Design review of the part built by this model. Coordinates are the model's own, in mm. A direction names the side the tool comes from. Round coordinates to 2 decimals unless told otherwise and drop trailing zeros. Loops run counter-clockwise (first coordinate to the right, second up) from the corner with the lowest first, then second, coordinate; pieces in that order, holes last. Notation, with made-up numbers: (-21.5, 88.25) - (17.5, 88.25) arc R15 cw to (17.5, 95.25) - close; hole circle Ø10 at (-14, -38.5). An arc over 180 degrees is marked (long way). Return JSON: item names as keys, results as strings. Group by question number.
from build123d import *

# Parameters (mm, degrees)
SKETCH3_R           = 2.5
BOSS_EXTRUDE1_DEPTH = 4.15
SKETCH4_R           = 1.5
BOSS_EXTRUDE2_DEPTH = 2
SKETCH4_3_R         = 1.5
BOSS_EXTRUDE3_DEPTH = 2
SKETCH4_5_R         = 1.5
BOSS_EXTRUDE4_DEPTH = 4.15
BOSS_EXTRUDE5_DEPTH = 2
CIRPATTERN1_COUNT   = 32


with BuildPart() as part:
    # Sketch3 → Boss-Extrude1 (new body)
    with BuildSketch(Plane(origin=(0, 0, 0), x_dir=(1, 0, 0), z_dir=(0, 1, 0))):
        with Locations(Location((0, 0, 0), (0, 0, 90))):
            Circle(SKETCH3_R)
    extrude(amount=BOSS_EXTRUDE1_DEPTH)

    # Sketch4 → Boss-Extrude2 (add)
    with BuildSketch(Plane(origin=(0, 4.15, 0), x_dir=(1, 0, 0), z_dir=(0, 1, 0))):
        with BuildLine():
            Line((30, 4), (10.915155748, 4))
            ThreePointArc((10.915155748, 4), (-11.625, 0), (10.915155748, -4))
            Line((10.915155748, -4), (30, -4))
            ThreePointArc((30, -4), (34, 0), (30, 4))
        make_face()
        with Locations(Location((30, 0, 0), (0, 0, 270))):
            Circle(SKETCH4_R, mode=Mode.SUBTRACT)
    extrude(amount=BOSS_EXTRUDE2_DEPTH)

    # Sketch4<3> → Boss-Extrude3 (add)
    with BuildSketch(Plane(origin=(0, 4.15, 0), x_dir=(1, 0, 0), z_dir=(0, 1, 0))):
        with Locations((30, 0)):
            Circle(SKETCH4_3_R)
    extrude(amount=BOSS_EXTRUDE3_DEPTH)

    # Sketch4<5> → Boss-Extrude4 (add)
    with BuildSketch(Plane(origin=(0, 4.15, 0), x_dir=(1, 0, 0), z_dir=(0, 1, 0))):
        with Locations(Location((30, 0, 0), (0, 0, 270))):
            Circle(SKETCH4_5_R)
    extrude(amount=-BOSS_EXTRUDE4_DEPTH)

    # Sketch7 → Boss-Extrude5 (add)
    with BuildSketch(Plane(origin=(0, 6.15, 0), x_dir=(1, 0, 0), z_dir=(0, 1, 0))):
        Polygon((-11.366268694, 0.75), (-11.366268694, -0.75), (-13.166268694, -0.25), (-13.166268694, 0.25), align=None)
    boss_extrude5 = extrude(amount=-BOSS_EXTRUDE5_DEPTH)

    # CirPattern1: Boss-Extrude5 ×32 about axis
    cirpattern1_axis = Axis((0, 0, 0), (0, 1, 0))
    for i in range(1, CIRPATTERN1_COUNT):
        add(boss_extrude5.rotate(cirpattern1_axis, i * 360 / CIRPATTERN1_COUNT))


solid = part.part
Q1. Draft analysis for pull direction X (two halves, no side actions). For faces 1 (the flat face through (8.418, 5.164, -9.082)), 2 (the flat face through (0, 0, 0)), 3 (the flat face through (-12.045, 5.164, 2.875)), state which applies: pulls with the +X half, pulls with the -X half, needs draft (parallel to the pull), parting line crosses it, or undercut.
Q2. Insertion check: pin 1 Ø2 at (x, y) = (19, 5.5) entering from -Z; pin 2 Ø3 at (y, z) = (4, -6) entering from +X; pin 3 Ø1.5 at (x, z) = (2, -5) entering from -Y. Each pin has a flat end and moves straight along its axis. Give the tip position at first contact, or say it passes through.
Q3. Add section B-B, the plane x = 18.5. State the section outline as (y, z) points, plus the area to 3 significant figures.
Q4. For line 1 (Z direction, x = 11.5, y = 5.5); line 2 (X direction, y = 4.5, z = -12); line 3 (X direction, y = 5.25, z = -10.5), list the stretches that pass through material, from the lowest coordinate up.
Q5. Add section A-A, the plane y = 1.25. State the section outline as (x, z) points.
Q6. Tool access review of faces 4 (the cylindrical face through (-11.123, 5.136, -3.381)), 5 (the flat face through (6.484, 5.164, -10.55)), 6 (the flat face through (1.964, 5.164, 12.249)), 7 (the flat face through (11.275, 5.164, 5.172)): name each direction out of +Z, -Z, +X, -X, +Y, -Y from which nothing blocks a thin tool from reaching the whole face with its end or side.
Evaluation:
{
 "1": {"face 1": "undercut", "face 2": "needs draft", "face 3": "pulls with the -X half"},
 "2": {"pin 1": "z = -4", "pin 2": "x = 12.26", "pin 3": "y = 4.15"},
 "3": {"outline": "(4.15, -4) - (6.15, -4) - (6.15, 4) - (4.15, 4) - close", "area": "16.0 mm²"},
 "4": {"line 1": "-5.2 to -4.21, -4 to 4, 4.21 to 5.2", "line 2": "-5.26 to -4.6, -2.88 to -1.84, -0.57 to 0.57, 1.84 to 2.88, 4.6 to 5.26", "line 3": "-7.42 to -6.43, -5.08 to 5.08, 6.43 to 7.42"},
 "5": {"outline": "circle Ø5 at (0, 0); circle Ø3 at (30, 0)"},
 "6": {"face 4": "-X, +Y, -Y", "face 5": "-Z, +Y, -Y", "face 6": "+Z, +Y, -Y", "face 7": "+Y, -Y"}
}
